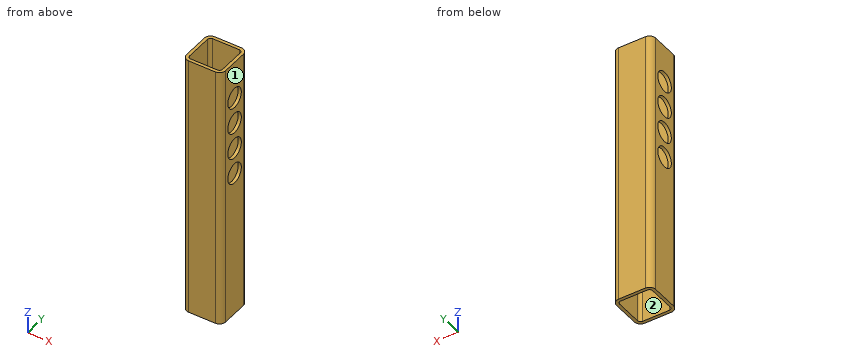
from build123d import *

# Parameters (mm, degrees)
EXTRUDE_1_DEPTH     = 170
SKETCH_2_R          = 6.5
CUT_EXTRUDE_1_DEPTH = 173.28247154


with BuildPart() as part:
    # Эскиз1 → Бобышка-Вытянуть1 (new body)
    with BuildSketch(Plane.XY):
        with BuildLine():
            Line((8.5, -12.5), (-8.5, -12.5))
            ThreePointArc((-8.5, -12.5), (-11.328427125, -11.328427125), (-12.5, -8.5))
            Line((-12.5, -8.5), (-12.5, 8.5))
            ThreePointArc((-12.5, 8.5), (-11.328427125, 11.328427125), (-8.5, 12.5))
            Line((-8.5, 12.5), (8.5, 12.5))
            ThreePointArc((8.5, 12.5), (11.328427125, 11.328427125), (12.5, 8.5))
            Line((12.5, 8.5), (12.5, -8.5))
            ThreePointArc((12.5, -8.5), (11.328427125, -11.328427125), (8.5, -12.5))
        make_face()
        with BuildLine():
            Line((-10.5, -8.5), (-10.5, 8.5))
            ThreePointArc((-10.5, 8.5), (-9.914213562, 9.914213562), (-8.5, 10.5))
            Line((-8.5, 10.5), (8.5, 10.5))
            ThreePointArc((8.5, 10.5), (9.914213562, 9.914213562), (10.5, 8.5))
            Line((10.5, 8.5), (10.5, -8.5))
            ThreePointArc((10.5, -8.5), (9.914213562, -9.914213562), (8.5, -10.5))
            Line((8.5, -10.5), (-8.5, -10.5))
            ThreePointArc((-8.5, -10.5), (-9.914213562, -9.914213562), (-10.5, -8.5))
        make_face(mode=Mode.SUBTRACT)
    extrude(amount=EXTRUDE_1_DEPTH)

    # Эскиз2 → Вырез-Вытянуть1 (cut, through all)
    with BuildSketch(Plane(origin=(12.5, 0, 0), x_dir=(0, 0, -1), z_dir=(1, 0, 0))):
        with Locations((-146, 0)):
            Circle(SKETCH_2_R)
        with Locations((-129, 0)):
            Circle(SKETCH_2_R)
        with Locations((-112, 0)):
            Circle(SKETCH_2_R)
        with Locations((-95, 0)):
            Circle(SKETCH_2_R)
    extrude(amount=-CUT_EXTRUDE_1_DEPTH, mode=Mode.SUBTRACT)


solid = part.part
Geometry check sheet. Reference: the model listing, model coordinates, mm. Face numbers are marked on the shaded views. A direction names the side the tool comes from. Round coordinates to 2 decimals unless told otherwise and drop trailing zeros. Loops run counter-clockwise (first coordinate to the right, second up) from the corner with the lowest first, then second, coordinate; pieces in that order, holes last. Notation, with made-up numbers: (-36, 42.25) - (20, 42.25) arc R23 ccw to (20, 67.25) - close; hole circle Ø3 at (16.5, 61). An arc over 180 degrees is marked (long way). One line per question, with ' | ' between items. Start each with the question number.
1. Cross-section at B-B on z = 146. Record the cut outline in (x, y).
2. Tool access check on the marked faces 1 and 2. Record the directions out of +Z, -Z, +X, -X, +Y, -Y that give a thin tool (end or side, any length) a straight path to the whole face; none if there is none.
3. Cross-section at C-C on y = -3.25. State how many separate pieces and enclosed holes the cut face has, then the cut area to 3 significant figures.
4. Cross-section at A-A on x = -2.25. Record the cut outline in (y, z).
5. Cross-section at D-D on z = 99. Record the cut outline in (x, y), then the cut area to 3 significant figures.
6. Scan lines: line 1 (X direction, y = 0.5, z = 50); line 2 (Y direction, x = 11.2, z = 95). Record each from-to range of solid material in increasing order. Write a range as [from, to].
Taken from the geometry:
1) outline: (-12.5, -8.5) arc R4 ccw to (-8.5, -12.5) - (8.5, -12.5) arc R4 ccw to (12.5, -8.5) - (12.5, -6.5) - (10.5, -6.5) - (10.5, -8.5) arc R2 cw to (8.5, -10.5) - (-8.5, -10.5) arc R2 cw to (-10.5, -8.5) - (-10.5, -6.5) - (-12.5, -6.5) - close; (-12.5, 6.5) - (-10.5, 6.5) - (-10.5, 8.5) arc R2 cw to (-8.5, 10.5) - (8.5, 10.5) arc R2 cw to (10.5, 8.5) - (10.5, 6.5) - (12.5, 6.5) - (12.5, 8.5) arc R4 ccw to (8.5, 12.5) - (-8.5, 12.5) arc R4 ccw to (-12.5, 8.5) - close
2) face 1: +Z, -Z, +X, +Y, -Y | face 2: +Z, -Z
3) separate pieces: 10 | enclosed holes: 0 | area: 500 mm²
4) outline: (-12.5, 0) - (-10.5, 0) - (-10.5, 170) - (-12.5, 170) - close; (10.5, 0) - (12.5, 0) - (12.5, 170) - (10.5, 170) - close
5) outline: (-12.5, -8.5) arc R4 ccw to (-8.5, -12.5) - (8.5, -12.5) arc R4 ccw to (12.5, -8.5) - (12.5, -5.12) - (10.5, -5.12) - (10.5, -8.5) arc R2 cw to (8.5, -10.5) - (-8.5, -10.5) arc R2 cw to (-10.5, -8.5) - (-10.5, -5.12) - (-12.5, -5.12) - close; (-12.5, 5.12) - (-10.5, 5.12) - (-10.5, 8.5) arc R2 cw to (-8.5, 10.5) - (8.5, 10.5) arc R2 cw to (10.5, 8.5) - (10.5, 5.12) - (12.5, 5.12) - (12.5, 8.5) arc R4 ccw to (8.5, 12.5) - (-8.5, 12.5) arc R4 ccw to (-12.5, 8.5) - close | area: 133 mm²
6) line 1: [-12.5, -10.5], [10.5, 12.5] | line 2: [-11.45, -6.5], [6.5, 11.45]
